Read the model definition and answer for the solid it produces. Units are mm, in the model's axes. A direction names the side the tool comes from. Give positions to 0.01 mm unless a question says otherwise; leave off trailing zeros. Loops run counter-clockwise (first coordinate to the right, second up) from the corner with the lowest first, then second, coordinate; pieces in that order, holes last. Notation, with made-up numbers: (89, 49) - (138, 49) arc R23 ccw to (138, 76) - close; hole circle Ø10 at (-31, 66.5). An arc over 180 degrees is marked (long way). Write item = value, one per line. Start each with the question number.
from build123d import *

# Parameters (mm, degrees)
F0_W     = 80
F0_H     = 60
F1_DEPTH = 20
F2_T     = -2
F3_W     = 77.999998
F3_H     = 57.999998
F4_DEPTH = 2


with BuildPart() as f1:
    # F0 (on Top) → F1 (new body)
    with BuildSketch(Plane.XY):
        Rectangle(F0_W, F0_H)
    extrude(amount=-F1_DEPTH)

    # F2
    f2_openings = [f1.faces().sort_by_distance(p)[0] for p in [
        (0, 0, -20),
    ]]
    offset(amount=F2_T, openings=f2_openings)

    # F3 (on face) → F4 (cut)
    with BuildSketch(Plane(origin=(0, 0, -20), x_dir=(1, 0, 0), z_dir=(0, 0, -1))):
        Rectangle(F3_W, F3_H)
    extrude(amount=-F4_DEPTH, mode=Mode.SUBTRACT)


solid = f1.part
1. A tool of negligible diameter and unlimited length cuts with its end or side. For faces 1 (the flat face through (-1, 30, -10)), 2 (the flat face through (-1, -28, -10)), from which of +Z, -Z, +X, -X, +Y, -Y can it reach the whole face along a straight path? Write none if from no direction.
2. For a pull along X with two mould halves and no side action, classify faces 3 (the flat face through (-39, 0, -19)), 4 (the flat face through (40, 0, -10)), 5 (the flat face through (-1, 0, 0)) as released by +X, released by -X, zero draft, split by the parting line, or undercut.
3. A cutting plane is placed at B-B on x = 23. Give the vertices of the cut face in (y, z).
4. Given P1, Ø3, axis at x = -16, y = 8, coming from the -Z side, flat-ended and moving along its own axis, determine where the tip first touches the part or whether it passes through.
5. A cutting plane is placed at A-A on z = -6. Give the vertices of the cut face in (x, y).
6. A cutting plane is placed at C-C on y = -26. Give the vertices of the cut face in (x, z).
7. Consider line 1 along Y through (x, z) = (-10, -11.25); line 2 along X through (y, z) = (13.5, -17.5); line 3 along Y through (x, z) = (16.5, -18.5). Determine where each line is inside the solid, lowest interval first. Write a range as [from, to].
Reply:
q1.face_1 = +Z, -Z, +X, -X, +Y
q1.face_2 = -Z
q2.face_3 = undercut
q2.face_4 = released by +X
q2.face_5 = zero draft
q3.outline = (-30, -20) - (-29, -20) - (-29, -18) - (-28, -18) - (-28, -2) - (28, -2) - (28, -18) - (29, -18) - (29, -20) - (30, -20) - (30, 0) - (-30, 0) - close
q4.P1 = -2
q5.outline = (-40, -30) - (40, -30) - (40, 30) - (-40, 30) - close; hole (-38, -28) - (38, -28) - (38, 28) - (-38, 28) - close
q6.outline = (-40, -20) - (-39, -20) - (-39, -18) - (-38, -18) - (-38, -2) - (38, -2) - (38, -18) - (39, -18) - (39, -20) - (40, -20) - (40, 0) - (-40, 0) - close
q7.line_1 = [-30, -28], [28, 30]
q7.line_2 = [-40, -38], [38, 40]
q7.line_3 = [-30, -29], [29, 30]
